```python
from build123d import *

# Parameters (mm, degrees)
F0_R     = 4
F1_DEPTH = 5.25
F2_R     = 3


with BuildPart() as f1:
    # F0 (on Front) → F1 (new body)
    with BuildSketch(Plane.XZ):
        Polygon((8.442299, 13), (0, 0), (37, 0), (28.557701, 13), align=None)
        with Locations((18.5, 6.5)):
            Circle(F0_R, mode=Mode.SUBTRACT)
    extrude(amount=F1_DEPTH)

    # F2
    f2_edges = [f1.edges().sort_by_distance(p)[0] for p in [
        (8.442299, -2.625, 13),
        (28.557701, -2.625, 13),
    ]]
    fillet(f2_edges, radius=F2_R)


solid = f1.part
```
Here's how the part is built. I have some questions about the finished solid (model axes, mm). Round coordinates to 2 decimals unless told otherwise and drop trailing zeros. Loops run counter-clockwise (first coordinate to the right, second up) from the corner with the lowest first, then second, coordinate; pieces in that order, holes last. Notation, with made-up numbers: (6.5, -8.75) -> (57.5, -8.75) arc R21 cw to (57.5, -4.75) -> close; hole circle Ø1 at (25, -39). An arc over 180 degrees is marked (long way). Answer as CSV lines item,"result".
1. For pin 1 (3 mm diameter, centred on y = -3.5, z = 6, fed in from +X), with a flat end and sliding along its axis, tell me the tip position at first contact or that it passes through.
Final values:
pin 1,"stops at x = 34.08"
2. If we section it at C-C on z = 6.5: Please give me the cut outline in (x, y).
Final values:
outline,"(4.22, -5.25) -> (14.5, -5.25) -> (14.5, 0) -> (4.22, 0) -> close; (22.5, -5.25) -> (32.78, -5.25) -> (32.78, 0) -> (22.5, 0) -> close"
3. If we section it at D-D on x = 9: Please give me the cut outline in (y, z).
Final values:
outline,"(-5.25, 0) -> (0, 0) -> (0, 12.8) -> (-5.25, 12.8) -> close"
4. If we section it at B-B on y = -3.2: Please give me the cut outline in (x, z), plus the area to 3 significant figures.
Final values:
outline,"(0, 0) -> (37, 0) -> (29.44, 11.63) arc R3 ccw to (26.93, 13) -> (10.07, 13) arc R3 ccw to (7.56, 11.63) -> close; hole circle Ø8 at (18.5, 6.5)"
area,"320 mm^2"
5. Thinking about a two-plate mould opening in X: for faces 1 (the face through (19, -3, 13)), 2 (the face through (3.83, -2.59, 5.9)), 3 (the face through (15.3, -2.6, 4.1)), which applies, released by +X, released by -X, zero draft, split by the parting line, or undercut?
Final values:
face 1,"zero draft"
face 2,"released by -X"
face 3,"undercut"
6. If we section it at A-A on x = 18.5: Please give me the cut outline in (y, z).
Final values:
outline,"(-5.25, 0) -> (0, 0) -> (0, 2.5) -> (-5.25, 2.5) -> close; (-5.25, 10.5) -> (0, 10.5) -> (0, 13) -> (-5.25, 13) -> close"
7. If I drill on L1, parallel to Z at x = 18.5, y = -3; L2, parallel to X at y = -4.1, z = 9.75; L3, parallel to Z at x = 21.5, y = -2.15, over which ranges is the centre line in solid material (lowest first)?
Final values:
L1,"z = 0 to 2.5, 10.5 to 13"
L2,"x = 6.33 to 16.17, 20.83 to 30.67"
L3,"z = 0 to 3.85, 9.15 to 13"
